Autodesk Inventor part; units mm, degrees
ref_plane "Start Plane" through (0, 0, 19.05) normal (0, 0, 1) x (1, 0, 0)
ref_plane "End Plane" through (0, 0, 323.85) normal (0, 0, 1) x (1, 0, 0)
ref_plane "Work Plane5" through (0, -19.05, 19.05) normal (0, 0, -1) x (-1, 0, 0)
ref_plane "Start Plane" through (0, 0, 19.05) normal (0, 0, 1) x (1, 0, 0)
ref_plane "End Plane" through (0, 0, 323.85) normal (0, 0, 1) x (1, 0, 0)
sketch "Sketch" plane through (0, 0, 0) normal (0, 0, 1) x (1, 0, 0)
  line L0 (-19.05, 19.05) -> (19.05, 19.05)
  line L1 (19.05, 19.05) -> (19.05, -19.05)
  line L2 (19.05, -19.05) -> (-19.05, -19.05)
  line L3 (-19.05, -19.05) -> (-19.05, 19.05)
  line L4 (15.875, 15.875) -> (-15.875, 15.875)
  line L5 (-15.875, 15.875) -> (-15.875, -15.875)
  line L6 (-15.875, -15.875) -> (15.875, -15.875)
  line L7 (15.875, -15.875) -> (15.875, 15.875)
  point P0 (0, 0)
  point P1 (0, 19.05)
  point P2 (-19.05, 0)
  dimension "width" = 38.1
  dimension "d1" = 3.175
extrude "Body" add sketch "Sketch" along normal up to surface (304.8 mm away) from surface at 19.05
sketch "Sketch4" plane through (0, 0, 0) normal (0, 0, 1) x (1, 0, 0)
  line L0 (0, 0) -> (10, 0)
ref_plane "Work Plane4" through (0, 0, 0) normal (0, -1, 0) x (1, 0, 0)
sketch "Sketch5" plane through (0, 0, 0) normal (0, -1, 0) x (1, 0, 0)
  line L0 (-2, 19.05) -> (12, 19.05)
  line L1 (-2, 323.85) -> (12, 323.85)
  dimension "d9" = 304.8
ref_plane "Work Plane5" through (0, -19.05, 19.05) normal (0, 0, -1) x (-1, 0, 0)
split "Split1" plane through (0, -19.05, 19.05) removes the side toward (0, 0, -1)
ref_plane "Work Plane6" through (723.9, 19.05, 323.85) normal (0, 0, 1) x (1, 0, 0)
split "Split2" plane through (723.9, 19.05, 323.85) removes the side toward (0, 0, 1)
equation "\"G_OFFSET_START\" = -19.05"
equation "\"G_OFFSET_END\" = 19.05"
equation "\"d4\" = -G_OFFSET_START"
equation "\"d5\" = length + G_OFFSET_END"
equation "\"G_L\" = 304.8"
properties part number "1.5x1.5x.125 Tube" material "Aluminum-6061"
Here's how the part is built. I have some questions about the finished solid (model axes, mm). A direction names the side the tool comes from. Give positions to 0.01 mm unless a question says otherwise; leave off trailing zeros. Order: outer loops, then holes, each group sorted by start corner. A loop starts at its lowest first (then second) coordinate and runs counter-clockwise, first axis right, second up. Notation, with made-up numbers: M 17,54.5 L 55,54.5 A22 ccw 55,69.5 Z; hole C -17.5,-8 d10. An arc over 180 degrees is marked long. Answer as a JSON object with one key per item and string values. Group by question number.
1) Please list where this line runs through material, in increasing order: L1, parallel to Y at x = 2.5, z = 153 (3 decimals). Write a range as [from, to].
2) Suppose I cut it at A-A, the plane x = -3.5. Write out the boundary of the cut face in (y, z) (3 decimals), plus the area to 3 significant figures.
3) We'd pull the mould along X, two halves only. Please class faces 3 (the flat face through (0, 15.875, 169)), 4 (the flat face through (0, -15.875, 169)), 5 (the flat face through (0, -19.05, 169)), 6 (the flat face through (19.05, 0, 169)): pulls with the +X half, pulls with the -X half, needs draft (parallel to the pull), parting line crosses it, or undercut.
4) On a 3-axis mill with a long thin cutter (end or side, diameter ignored), from which of +Z, -Z, +X, -X, +Y, -Y can I reach the whole of each face in a straight line? I mean faces 1 (the flat face through (15.875, 0, 169)), 2 (the flat face through (-17, 0, 323.85)). Say none if no direction works.
5) Suppose I cut it at C-C, the plane z = 296. Write out the boundary of the cut face in (x, y) (3 decimals).
Results found:
{
 "1": {"L1": "[-19.05, -15.875], [15.875, 19.05]"},
 "2": {"outline": "M -19.05,19.05 L -15.875,19.05 L -15.875,323.85 L -19.05,323.85 Z; M 15.875,19.05 L 19.05,19.05 L 19.05,323.85 L 15.875,323.85 Z", "area": "1,940 mm²"},
 "3": {"face 3": "undercut", "face 4": "undercut", "face 5": "needs draft", "face 6": "pulls with the +X half"},
 "4": {"face 1": "+Z, -Z", "face 2": "+Z, +X, -X, +Y, -Y"},
 "5": {"outline": "M -19.05,-19.05 L 19.05,-19.05 L 19.05,19.05 L -19.05,19.05 Z; hole M -15.875,-15.875 L 15.875,-15.875 L 15.875,15.875 L -15.875,15.875 Z"}
}
